from build123d import *

# Parameters (mm, degrees)
PAD_DEPTH            = 2
SKETCH002_R          = 6
PAD002_DEPTH         = 3
POCKET_DEPTH         = 3.001
SKETCH005_R          = 1.25
POCKET001_DEPTH      = 0.001
POCKET001_DEPTH_BACK = 3.001
POCKET002_DEPTH      = 2
SKETCH012_W          = 25
SKETCH012_H          = 50.4
SKETCH012_H_2        = 36.4
POCKET006_DEPTH      = 0.001
POCKET006_DEPTH_BACK = 3.001
SKETCH014_W          = 2
SKETCH014_H          = 50.4
PAD006_DEPTH         = 4
SKETCH015_W          = 2.4
SKETCH015_H          = 36.4
PAD007_DEPTH         = 3
SKETCH018_R          = 2.9
POCKET008_DEPTH      = 1.5
PAD010_DEPTH         = 4
SKETCH024_R          = 1.25
POCKET010_DEPTH      = 0.001
POCKET010_DEPTH_BACK = 6.001
SKETCH032_W          = 20
SKETCH032_H          = 50
POCKET016_DEPTH      = 0.001
POCKET016_DEPTH_BACK = 6.001
SKETCH041_W          = 15
SKETCH041_H          = 5.8
SKETCH041_H_2        = 3
POCKET020_DEPTH      = 0.001
POCKET020_DEPTH_BACK = 6.001


with BuildPart() as part:
    # Sketch → Pad (new body)
    with BuildSketch(Plane.XY):
        with BuildLine():
            Line((-29.5, -64), (29.5, -64))
            ThreePointArc((29.5, -64), (31.267767, -63.267767), (32, -61.5))
            Line((32, -42.5), (32, -61.5))
            ThreePointArc((34.5, -40), (32.732233, -40.732233), (32, -42.5))
            Line((34.5, 12), (34.5, -40))
            ThreePointArc((32, 14.5), (32.732233, 12.732233), (34.5, 12))
            Line((32, 21.5), (32, 14.5))
            ThreePointArc((32, 21.5), (31.267767, 23.267767), (29.5, 24))
            Line((29.5, 24), (-34.5, 24))
            ThreePointArc((-34.5, 24), (-36.267767, 23.267767), (-37, 21.5))
            Line((-37, 21.5), (-37, -40))
            ThreePointArc((-37, -40), (-36.267767, -41.767767), (-34.5, -42.5))
            ThreePointArc((-32, -45), (-32.732233, -43.232233), (-34.5, -42.5))
            Line((-32, -45), (-32, -61.5))
            ThreePointArc((-32, -61.5), (-31.267767, -63.267767), (-29.5, -64))
        make_face()
    extrude(amount=PAD_DEPTH)

    # Sketch002 → Pad002 (join)
    with BuildSketch(Plane.XY):
        with Locations((-23.25, -55)):
            Circle(SKETCH002_R)
        with Locations((23.25, -55)):
            Circle(SKETCH002_R)
        with Locations((-23.25, -10)):
            Circle(SKETCH002_R)
        with Locations((23.25, -10)):
            Circle(SKETCH002_R)
    extrude(amount=PAD002_DEPTH)

    # Sketch004 → Pocket (cut, through all)
    with BuildSketch(Plane.XY):
        Polygon((-21, 18.3), (-21, 5.3), (21, 5.3), (21, -3.7), (28, -3.7), (28, 18.3), align=None)
    extrude(amount=POCKET_DEPTH, mode=Mode.SUBTRACT)

    # Sketch005 → Pocket001 (cut, two sides)
    with BuildSketch(Plane.XY) as pocket001_sk:
        with Locations((-23.25, -10)):
            Circle(SKETCH005_R)
        with Locations((23.25, -10)):
            Circle(SKETCH005_R)
        with Locations((-23.25, -55)):
            Circle(SKETCH005_R)
        with Locations((23.25, -55)):
            Circle(SKETCH005_R)
    extrude(amount=-POCKET001_DEPTH, mode=Mode.SUBTRACT)
    extrude(pocket001_sk.sketch, amount=POCKET001_DEPTH_BACK, mode=Mode.SUBTRACT)

    # Sketch003 → Pocket002 (cut)
    with BuildSketch(Plane.XY):
        Polygon((-20.882864, -10), (-22.066432, -7.95), (-24.433568, -7.95), (-25.617136, -10), (-24.433568, -12.05), (-22.066432, -12.05), align=None)
        Polygon((25.617136, -10), (24.433568, -7.95), (22.066432, -7.95), (20.882864, -10), (22.066432, -12.05), (24.433568, -12.05), align=None)
        Polygon((-22.066432, -52.95), (-24.433568, -52.95), (-25.617136, -55), (-24.433568, -57.05), (-22.066432, -57.05), (-20.882864, -55), align=None)
        Polygon((24.433568, -52.95), (22.066432, -52.95), (20.882864, -55), (22.066432, -57.05), (24.433568, -57.05), (25.617136, -55), align=None)
    extrude(amount=POCKET002_DEPTH, mode=Mode.SUBTRACT)

    # Sketch012 → Pocket006 (cut, two sides)
    with BuildSketch(Plane.XY) as pocket006_sk:
        with Locations((-43.3, -8)):
            Rectangle(SKETCH012_W, SKETCH012_H)
        with Locations((43.3, -10)):
            Rectangle(SKETCH012_W, SKETCH012_H_2)
    extrude(amount=-POCKET006_DEPTH, mode=Mode.SUBTRACT)
    extrude(pocket006_sk.sketch, amount=POCKET006_DEPTH_BACK, mode=Mode.SUBTRACT)

    # Sketch014 (on Face5 of Pocket006) → Pad006 (join)
    with BuildSketch(Plane.XY.offset(2)):
        with Locations((-29.8, -8)):
            Rectangle(SKETCH014_W, SKETCH014_H)
    extrude(amount=PAD006_DEPTH)

    # Sketch015 (on Face5 of Pocket006) → Pad007 (join)
    with BuildSketch(Plane.XY.offset(2)):
        with Locations((29.6, -10)):
            Rectangle(SKETCH015_W, SKETCH015_H)
    extrude(amount=PAD007_DEPTH)

    # Sketch018 → Pocket008 (cut)
    with BuildSketch(Plane.XY):
        with Locations((-15, 21)):
            Circle(SKETCH018_R)
        with Locations((15, 21)):
            Circle(SKETCH018_R)
        with Locations((-15, -55)):
            Circle(SKETCH018_R)
        with Locations((15, -55)):
            Circle(SKETCH018_R)
    extrude(amount=POCKET008_DEPTH, mode=Mode.SUBTRACT)

    # Sketch020 (on Face5 of Pocket008) → Pad010 (join)
    with BuildSketch(Plane.XY.offset(2)):
        with BuildLine():
            Line((-34.5, 24), (29.5, 24))
            ThreePointArc((32, 21.5), (31.267767, 23.267767), (29.5, 24))
            Line((32, 21.5), (32, 14.5))
            ThreePointArc((32, 14.5), (32.732233, 12.732233), (34.5, 12))
            Line((34.5, 12), (34.5, 8.2))
            Line((29, 8.2), (34.5, 8.2))
            Line((29, 19), (29, 8.2))
            Line((-34, 19), (29, 19))
            Line((-34, 17.2), (-34, 19))
            Line((-37, 17.2), (-34, 17.2))
            Line((-37, 21.5), (-37, 17.2))
            ThreePointArc((-34.5, 24), (-36.267767, 23.267767), (-37, 21.5))
        make_face()
        with BuildLine():
            Line((34.5, -28.2), (34.5, -40))
            ThreePointArc((34.5, -40), (32.732233, -40.732233), (32, -42.5))
            Line((32, -42.5), (32, -61.5))
            ThreePointArc((29.5, -64), (31.267767, -63.267767), (32, -61.5))
            Line((29.5, -64), (-29.5, -64))
            ThreePointArc((-32, -61.5), (-31.267767, -63.267767), (-29.5, -64))
            Line((-32, -61.5), (-32, -45))
            ThreePointArc((-32, -45), (-32.732233, -43.232233), (-34.5, -42.5))
            ThreePointArc((-37, -40), (-36.267767, -41.767767), (-34.5, -42.5))
            Line((-37, -40), (-37, -33.2))
            Line((-34, -33.2), (-37, -33.2))
            Line((-34, -39.5), (-34, -33.2))
            Line((-29, -39.5), (-34, -39.5))
            Line((-29, -59), (-29, -39.5))
            Line((29, -59), (-29, -59))
            Line((29, -28.2), (29, -59))
            Line((34.5, -28.2), (29, -28.2))
        make_face()
    extrude(amount=PAD010_DEPTH)

    # Sketch024 → Pocket010 (cut, two sides)
    with BuildSketch(Plane.XY) as pocket010_sk:
        with Locations((-34, 21)):
            Circle(SKETCH024_R)
        with Locations((27.5, 21)):
            Circle(SKETCH024_R)
        with Locations((27.5, -61)):
            Circle(SKETCH024_R)
        with Locations((-27.5, -61)):
            Circle(SKETCH024_R)
    extrude(amount=-POCKET010_DEPTH, mode=Mode.SUBTRACT)
    extrude(pocket010_sk.sketch, amount=POCKET010_DEPTH_BACK, mode=Mode.SUBTRACT)

    # Sketch032 → Pocket016 (cut, two sides)
    with BuildSketch(Plane.XY) as pocket016_sk:
        with Locations((0, -25)):
            Rectangle(SKETCH032_W, SKETCH032_H)
    extrude(amount=-POCKET016_DEPTH, mode=Mode.SUBTRACT)
    extrude(pocket016_sk.sketch, amount=POCKET016_DEPTH_BACK, mode=Mode.SUBTRACT)

    # Sketch041 → Pocket020 (cut, two sides)
    with BuildSketch(Plane.XY) as pocket020_sk:
        with Locations((-27.5, -35.7)):
            Rectangle(SKETCH041_W, SKETCH041_H)
        with Locations((25.7, -29.5)):
            Rectangle(SKETCH041_W, SKETCH041_H_2)
    extrude(amount=-POCKET020_DEPTH, mode=Mode.SUBTRACT)
    extrude(pocket020_sk.sketch, amount=POCKET020_DEPTH_BACK, mode=Mode.SUBTRACT)


solid = part.part
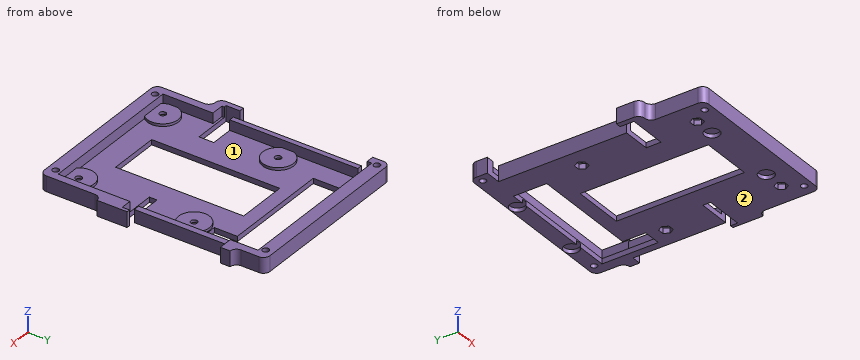
For this review, take the finished solid that the model builds, in its own axes (mm). Face numbers are marked on the shaded views. Round coordinates to 2 decimals unless told otherwise and drop trailing zeros. Loops run counter-clockwise (first coordinate to the right, second up) from the corner with the lowest first, then second, coordinate; pieces in that order, holes last. Notation, with made-up numbers: (73, 76) - (124, 76) arc R26 ccw to (124, 97) - close; hole circle Ø3 at (5, 51). An arc over 180 degrees is marked (long way). Use one line per item in the form item = value.
Item 1: Clearance check with flat-ended pins moving along their axes: P1, Ø1.7, axis at x = 15.5, y = 22.5, coming from the -Z side; P2, Ø2.5, axis at y = -2.5, z = 1.5, coming from the +X side; P3, Ø2, axis at y = -25, z = 3.5, coming from the -X side; P4, Ø4.5, axis at x = 24, y = -10, coming from the -Z side. State where each tip first meets the part, or that it passes through.
Answers:
P1 = 1.5
P2 = 30.8
P3 = -30.8
P4 = 0
Item 2: Mouldability with a two-part tool opening along X and no side actions: class the marked faces 1 and 2 as +X half, -X half, draft (parallel to the pull), parting line (faces both ways), or undercut.
Answers:
face_1 = undercut
face_2 = draft
Item 3: Consider section A-A on x = -8.5. Write out the cut boundary in (y, z).
Answers:
outline = (-64, 0) - (-50, 0) - (-50, 2) - (-59, 2) - (-59, 6) - (-64, 6) - close; (0, 0) - (5.3, 0) - (5.3, 2) - (0, 2) - close; (18.3, 0) - (24, 0) - (24, 6) - (19, 6) - (19, 2) - (18.3, 2) - close
Item 4: Consider section C-C on x = 23.25. State how many separate pieces and enclosed holes the cut face has, then the cut area to 3 significant figures.
Answers:
separate_pieces = 5
enclosed_holes = 0
area = 167 mm^2
Item 5: Consider section B-B on y = -29.5. Write out the cut boundary in (x, z).
Answers:
outline = (-30.8, 0) - (-10, 0) - (-10, 2) - (-28.8, 2) - (-28.8, 6) - (-30.8, 6) - close; (10, 0) - (18.2, 0) - (18.2, 2) - (10, 2) - close; (33.2, 0) - (34.5, 0) - (34.5, 6) - (33.2, 6) - close
Item 6: For line 1 (X direction, y = -30, z = 1.6); line 2 (Y direction, x = -27.5, z = 1.8); line 3 (Y direction, x = 23.25, z = 2.7), list the stretches that pass through material, from the lowest coordinate up.
Answers:
line_1 = -30.8 to -10, 10 to 18.2, 33.2 to 34.5
line_2 = -64 to -62.25, -59.75 to -38.6, -32.8 to 24
line_3 = -64 to -56.25, -53.75 to -49, -16 to -11.25, -8.75 to -4, 19 to 24
